from build123d import *

# Parameters (mm, degrees)
SKETCH1_W                               = 66
SKETCH1_H                               = 100
BOSS_EXTRUDE1_DEPTH                     = 5
SKETCH2_R                               = 6
BOSS_EXTRUDE2_DEPTH                     = 5
CBORE_FOR_M5_HEX_HEAD_BOLT1_D           = 5
CBORE_FOR_M5_HEX_HEAD_BOLT1_CBORE_D     = 8.2
CBORE_FOR_M5_HEX_HEAD_BOLT1_CBORE_DEPTH = 8
FILLET1_R                               = 2.5


with BuildPart() as part:
    # Sketch1 → Boss-Extrude1 (new body)
    with BuildSketch(Plane(origin=(0, 0, 0), x_dir=(1, 0, 0), z_dir=(0, 1, 0))):
        Rectangle(SKETCH1_W, SKETCH1_H)
    extrude(amount=BOSS_EXTRUDE1_DEPTH)

    # Sketch2 → Boss-Extrude2 (add)
    with BuildSketch(Plane(origin=(0, 5, 0), x_dir=(1, 0, 0), z_dir=(0, 1, 0))):
        with Locations(Location((-16, 35, 0), (0, 0, 270))):
            Circle(SKETCH2_R)
        with Locations(Location((16, 35, 0), (0, 0, 90))):
            Circle(SKETCH2_R)
        with Locations(Location((16, -35, 0), (0, 0, 270))):
            Circle(SKETCH2_R)
        with Locations(Location((-16, -35, 0), (0, 0, 90))):
            Circle(SKETCH2_R)
    extrude(amount=BOSS_EXTRUDE2_DEPTH)

    # CBORE for M5 Hex Head Bolt1 (through all)
    with Locations(Plane(origin=(0, 10, 0), x_dir=(1, 0, 0), z_dir=(0, 1, 0))):
        with Locations((-16, 35), (16, 35), (16, -35), (-16, -35)):
            CounterBoreHole(CBORE_FOR_M5_HEX_HEAD_BOLT1_D / 2, CBORE_FOR_M5_HEX_HEAD_BOLT1_CBORE_D / 2, CBORE_FOR_M5_HEX_HEAD_BOLT1_CBORE_DEPTH)

    # Fillet1
    fillet1_edges = [part.edges().sort_by_distance(p)[0] for p in [
        (-33, 2.5, -50),
        (33, 2.5, -50),
        (33, 2.5, 50),
        (-33, 2.5, 50),
    ]]
    fillet(fillet1_edges, radius=FILLET1_R)


solid = part.part
For this review, take the finished solid that the model builds, in its own axes (mm). A direction names the side the tool comes from. Round coordinates to 2 decimals unless told otherwise and drop trailing zeros. Loops run counter-clockwise (first coordinate to the right, second up) from the corner with the lowest first, then second, coordinate; pieces in that order, holes last. Notation, with made-up numbers: (-9, -1.5) - (16, -1.5) arc R18 ccw to (16, 4.5) - close; hole circle Ø8 at (-27, -14.75). An arc over 180 degrees is marked (long way). One line per item, written item: value. Start each with the question number.
Item 1: The part is to be moulded in two halves that separate along Z. For faces 1 (the flat face through (0, 2, -50)), 2 (the flat face through (13, 10, 39)), 3 (the flat face through (0, 5, -1)), say which applies: +Z half, -Z half, draft (parallel to the pull), parting line (faces both ways), or undercut.
Item 2: Take a section at A-A (y = 7.25). Give the boundary of the cut face in (x, z).
Item 3: Take a section at B-B (x = 16). Give the boundary of the cut face in (y, z), plus the area to 3 significant figures.
Item 4: Take a section at C-C (z = -35). Give the boundary of the cut face in (x, y).
Item 5: Take a section at D-D (z = 6.5). Give the boundary of the cut face in (x, y).
Item 6: Clearance check with flat-ended pins moving along their axes: pin 1 Ø7.5 at (x, z) = (-16, -35) entering from +Y; pin 2 Ø2.5 at (x, z) = (15.5, 34) entering from +Y. State where each tip first meets the part, or that it passes through.
Item 7: For L1, parallel to X at y = 1.3, z = 35; L2, parallel to X at y = 7.25, z = 35; L3, parallel to Z at x = -16, y = 1.6, list the stretches that pass through material, from the lowest coordinate up.
Item 8: For faces 4 (the cylindrical face through (-14.16, 0.99, 33.31)), 5 (the flat face through (-18, 2, 37)), list the 3-axis set-ups (+Z, -Z, +X, -X, +Y, -Y) from which the entire face can be reached by the end or side of a thin tool; tool diameter is ignored.
Answer below:
1. face 1: -Z half
1. face 2: draft
1. face 3: undercut
2. outline: circle Ø12 at (-16, -35); circle Ø12 at (-16, 35); circle Ø12 at (16, -35); circle Ø12 at (16, 35); hole circle Ø8.2 at (-16, -35); hole circle Ø8.2 at (-16, 35); hole circle Ø8.2 at (16, -35); hole circle Ø8.2 at (16, 35)
3. outline: (0, -50) - (5, -50) - (5, -41) - (10, -41) - (10, -39.1) - (2, -39.1) - (2, -37.5) - (0, -37.5) - close; (0, -32.5) - (2, -32.5) - (2, -30.9) - (10, -30.9) - (10, -29) - (5, -29) - (5, 29) - (10, 29) - (10, 30.9) - (2, 30.9) - (2, 32.5) - (0, 32.5) - close; (0, 37.5) - (2, 37.5) - (2, 39.1) - (10, 39.1) - (10, 41) - (5, 41) - (5, 50) - (0, 50) - close
3. area: 469 mm2
4. outline: (-33, 0) - (-18.5, 0) - (-18.5, 2) - (-20.1, 2) - (-20.1, 10) - (-22, 10) - (-22, 5) - (-33, 5) - close; (-13.5, 0) - (13.5, 0) - (13.5, 2) - (11.9, 2) - (11.9, 10) - (10, 10) - (10, 5) - (-10, 5) - (-10, 10) - (-11.9, 10) - (-11.9, 2) - (-13.5, 2) - close; (18.5, 0) - (33, 0) - (33, 5) - (22, 5) - (22, 10) - (20.1, 10) - (20.1, 2) - (18.5, 2) - close
5. outline: (-33, 0) - (33, 0) - (33, 5) - (-33, 5) - close
6. pin 1: stops at y = 2
6. pin 2: passes through
7. L1: x = -33 to -18.5, -13.5 to 13.5, 18.5 to 33
7. L2: x = -22 to -20.1, -11.9 to -10, 10 to 11.9, 20.1 to 22
7. L3: z = -50 to -37.5, -32.5 to 32.5, 37.5 to 50
8. face 4: +Y, -Y
8. face 5: +Y
